Model file for the job. Use its own axes, mm. A direction names the side the tool comes from. Round coordinates to 2 decimals unless told otherwise and drop trailing zeros. Loops run counter-clockwise (first coordinate to the right, second up) from the corner with the lowest first, then second, coordinate; pieces in that order, holes last. Notation, with made-up numbers: (-13.5, 33.25) - (-8.5, 33.25) arc R19 cw to (-8.5, 37.25) - close; hole circle Ø8 at (-10.75, -5). An arc over 180 degrees is marked (long way). Answer as a JSON object with one key per item and string values.
Autodesk Inventor part; units mm, degrees
ref_plane "Work Plane1" through (10.95, 0, 0) normal (0, 0, -1) x (1, 0, 0)
ref_plane "YZ Plane" through (0, 0, 0) normal (1, 0, 0) x (0, 1, 0)
ref_plane "XZ Plane" through (0, 0, 0) normal (0, 1, 0) x (-1, 0, 0)
sketch "Sketch1" plane through (0, 0, 0) normal (0, 0, 1) x (1, 0, 0)
  line L0 (-4.4577, 0) -> (-4.4577, 6.0778)
  line L1 (0, 8.763) -> (0, 4.7625)
  line L2 (31.75, 4.7625) -> (57.15, 4.7625)
  line L3 (57.15, 4.7625) -> (57.15, 0)
  line L4 (57.15, 0) -> (-4.4577, 0)
  arc A0 (0, 8.763) -> (-2.9052, 9.4071) centre (-1.524, 8.763) ccw
  line L5 (0, -2.1146) -> (0, 12.6875)
  line L6 (-16.7792, 0) -> (69.4715, 0)
  line L7 (0, 4.7625) -> (0.0001, 4.7625)
  line L8 (0.0001, 4.7625) -> (0.0001, 4.7625)
  line L9 (0.0001, 4.7625) -> (20.6248, 4.7625)
  line L10 (20.6248, 4.7625) -> (31.75, 4.7625)
  line L11 (-4.4577, 6.0778) -> (-2.9052, 9.4071)
  line L12 (0.0001, 4.7625) -> (31.75, 4.7625) construction
  line L13 (31.75, 4.7625) -> (31.75, 0) construction
  dimension "d0" = 1.524
  dimension "d1" = 57.15
  dimension "d2" = 25.4
  dimension "d3" = 20.574
  dimension "d4" = 9.525
  dimension "d5" = 4.4577
  dimension "d15" = 9.525
  dimension "d16" = 9.525
  dimension "d17" = 0.0001
  dimension "d18" = 11.1252
  dimension "d19" = 25
revolve "Body" add sketch "Sketch1" angle 360 about axis through (57.15, 0, 0) along (-1, 0, 0)
sketch "Sketch2" plane through (0, 0, 0) normal (1, 0, 0) x (0, 0, -1)
  line L0 (7.1438, 4.1244) -> (7.1437, -4.1244)
  line L1 (7.1437, -4.1244) -> (0, -8.2489)
  line L2 (0, -8.2489) -> (-7.1438, -4.1244)
  line L3 (-7.1438, -4.1244) -> (-7.1437, 4.1244)
  line L4 (-7.1437, 4.1244) -> (0, 8.2489)
  line L5 (0, 8.2489) -> (7.1438, 4.1244)
  point P0 (0, 0)
  point P1 (0, 0)
  dimension "d23" = 14.2875
extrude "Head" add sketch "Sketch2" against normal blind 9.906
sketch "Sketch3" plane through (0, 0, 0) normal (0, 0, 1) x (1, 0, 0)
  line L0 (-9.906, 7.1437) -> (-9.906, 8.2489)
  line L1 (-9.906, 8.2489) -> (-9.2679, 8.2489)
  line L2 (-9.2679, 8.2489) -> (-9.906, 7.1437)
  line L3 (-11.1981, 0) -> (-2.1531, 0)
  line L4 (-9.906, 8.2489) -> (-9.906, 4.1244)
  line L5 (-3.4453, 8.2489) -> (-9.906, 8.2489)
  point P0 (-9.906, 4.1244)
  dimension "d8" = 30
  dimension "d22" = 14.2875
revolve "Chamfer1" cut sketch "Sketch3" angle 360 about axis through (-10, 0, 0) along (1, 0, 0)
thread "Thread"
chamfer "Chamfer2" distance 0.9739 distance2 0.9739 1 edges at (57.15, -4.7625, 0) measured on face at (57.15, 0.5629, 1.4843)
ref_plane "Work Plane1" through (10.95, 0, 0) normal (0, 0, -1) x (1, 0, 0)
equation "\"d23\" = SW"
equation "\"d6\" = KOH"
equation "\"d10\" = GEL"
equation "\"d13\" = -0.5 * SPD + 0.5 * GD"
equation "\"d14\" = GUL"
equation "\"d0\" = PHH"
equation "\"d1\" = NLG"
equation "\"d2\" = GEL"
equation "\"d3\" = LADI"
equation "\"d4\" = GD"
equation "\"d5\" = 0.45 * KOH"
equation "\"d15\" = SD2"
equation "\"d16\" = BDM"
equation "\"d18\" = GAL"
equation "\"d19\" = KEWI"
equation "\"d8\" = ANG1"
equation "\"d22\" = SW0"
equation "\"NLG\" = 57.15"
equation "\"GD\" = NND"
equation "\"BDM\" = NND"
equation "\"KOH\" = 9.906"
equation "\"GEL\" = 25.4"
equation "\"LADI\" = 20.574"
equation "\"SW\" = 14.2875"
equation "\"PHH\" = 1.524"
equation "\"SW0\" = SW"
equation "\"SPD\" = 7.5773"
equation "\"SD2\" = NND"
equation "\"SD\" = 0"
equation "\"ANG1\" = 30deg"
equation "\"KEWI\" = 25deg"
equation "\"GAL\" = 11.1252"
equation "\"GUL\" = 0.97385"
equation "\"THREADDIA\" = 9.525"
equation "\"SDH\" = SW"
equation "\"TOA\" = 30deg"
equation "\"NND\" = 9.525"
equation "\"E0\" = 1.155 * SW"
equation "\"GD1\" = 7.5773"
properties part number "92979A186" material "Steel, Mild"
1) Slice it at A-A on x = 1. List the corners of the cut face in (y, z) (1 decimal).
Values follow:
{"outline": "circle Ø9.5 at (0, 0)"}
2) Drop flat-ended pins along their axis: P1, Ø6, axis at x = 0, z = 6, coming from the -Y side; P2, Ø5, axis at y = 2, z = -5.5, coming from the +X side; P3, Ø10, axis at x = 26, y = -4, coming from the -Z side; P4, Ø10, axis at x = 43.5, z = 7.5, coming from the +Y side. Give the stop position or say it passes through.
Values follow:
{"P1": "y = -9.73", "P2": "x = 57.15", "P3": "z = -4.76", "P4": "y = 4.05"}
3) Probe probe 1 along Y at (x, z) = (39, 0.25); probe 2 along X at (y, z) = (5.25, -2.75); probe 3 along Y at (x, z) = (32.5, 2). List the from-to ranges inside material, lowest first.
Values follow:
{"probe 1": "-4.76 to 4.76", "probe 2": "-9.91 to 0", "probe 3": "-4.32 to 4.32"}
4) Tool access for faces 1 (the flat face through (-6.63, 6.16, 3.62)), 2 (the flat face through (-6.63, -6.216, 3.522)), 3 (the flat face through (-6.63, -6.16, -3.62)), 4 (the flat face through (-6.63, 6.216, -3.522)), 5 (the flat face through (0, 4, 4)): list every direction of +Z, -Z, +X, -X, +Y, -Y with a clear straight run to the whole face (end or side of a thin tool).
Values follow:
{"face 1": "+Z, -X, +Y", "face 2": "+Z, -X, -Y", "face 3": "-Z, -X, -Y", "face 4": "-Z, -X, +Y", "face 5": "+X"}
